```python
from build123d import *

# Parameters (mm, degrees)
F0_R     = 7.5
F1_DEPTH = 50
F3_DEPTH = 12.5
F4_W     = 15
F4_H     = 7.736891
F4_H_2   = 4.14352
F5_DEPTH = 15
F6_R     = 2
F7_DEPTH = 12.5


with BuildPart() as f1:
    # F0 (on Front) → F1 (new body)
    with BuildSketch(Plane.XZ):
        Circle(F0_R)
    extrude(amount=F1_DEPTH)

    # F2 (on Right) → F3 (cut, symmetric)
    with BuildSketch(Plane.YZ):
        Polygon((-44.571992, 11.14893), (-51.264416, 11.14893), (-51.264416, -8.581314), (-47.007408, -8.41625), (-48.95056, -5.98029), (-47.531635, -4.853975), (-43.883123, -4.709495), (-48.910081, -2.602493), (-46.984833, -0.98913), (-49.004711, 1.153992), (-42.819649, 1.551311), (-48.76826, 3.143417), (-46.388377, 4.090473), (-48.69375, 6.484859), align=None)
    extrude(amount=F3_DEPTH, both=True, mode=Mode.SUBTRACT)

    # F4 (on Front) → F5 (cut)
    with BuildSketch(Plane.XZ):
        with Locations((-0.000368, -8.868445)):
            Rectangle(F4_W, F4_H)
        with Locations((0.000368, 7.07176)):
            Rectangle(F4_W, F4_H_2)
    extrude(amount=F5_DEPTH, mode=Mode.SUBTRACT)

    # F6 (on Right) → F7 (cut, symmetric)
    with BuildSketch(Plane.YZ):
        with Locations((-7.5, 0)):
            Circle(F6_R)
    extrude(amount=F7_DEPTH, both=True, mode=Mode.SUBTRACT)


solid = f1.part
```
Build history of the part. All positions in model axes, mm. A direction names the side the tool comes from. Coordinates: 2 decimals unless noted, no trailing zeros. Order: outer loops, then holes, each group sorted by start corner. A loop starts at its lowest first (then second) coordinate and runs counter-clockwise, first axis right, second up. Notation, with made-up numbers: (38.5, 64.25) -> (93.5, 64.25) arc R31 cw to (93.5, 93.25) -> close; hole circle Ø3 at (4, 70). An arc over 180 degrees is marked (long way). Answer in a Markdown table with one row per item. Add a question column.
Q1. Band-saw the part on D-D, the plane y = -35. List the corners of the cut face in (x, z).
Q2. Which spindle directions (+Z, -Z, +X, -X, +Y, -Y) get a long thin tool onto all of the face, cutting with end or side? Do faces 5 (the face through (0, -7, -5)), 6 (the face through (0.104, -47.961, -1.807)), 7 (the face through (0.06, -48.47, -6.58)), 8 (the face through (0, -15, 6)). Say none if no direction does.
Q3. Band-saw the part on A-A, the plane x = 0. List the corners of the cut face in (y, z).
Q4. Band-saw the part on C-C, the plane z = 0. List the corners of the cut face in (x, y).
Q5. Band-saw the part on B-B, the plane y = -6.5. List the corners of the cut face in (x, z).
Q6. Drop flat-ended pins along their axis: pin 1 (3 mm diameter, centred on x = -5.5, z = 0, fed in from +Y); pin 2 (5 mm diameter, centred on y = -39, z = -5.5, fed in from +X); pin 3 (1 mm diameter, centred on x = 3.5, z = -5, fed in from -Y); pin 4 (1.5 mm diameter, centred on x = 1.5, z = -0.5, fed in from -Y). Give the stop position or say it passes through.
Q7. Wall check: line 1 along Z through (x, y) = (0.75, -7.5); line 2 along Z through (x, y) = (1, -12.5); line 3 along Z through (x, y) = (-5, -33.5). Give the ranges that are in metal, low to high. Write a range as [from, to].
Q8. Mould opens along Z. For faces 1 (the face through (0.053, -48.351, 6.873)), 2 (the face through (0.105, -9.498, 0.088)), 3 (the face through (3.461, -29.604, -6.654)), 4 (the face through (0, 0, 0)) say: +Z half, -Z half, draft (parallel to the pull), parting line (faces both ways), or undercut.
Answers follow:
| question | item | result |
|---|---|---|
| 1 | outline | circle Ø15 at (0, 0) |
| 2 | face 5 | -Z, +X, -X, +Y |
| 2 | face 6 | +X, -X, -Y |
| 2 | face 7 | -Z, +X, -X, -Y |
| 2 | face 8 | +Z, +X, -X, +Y |
| 3 | outline | (-49, 1.15) -> (-46.98, -0.99) -> (-48.91, -2.6) -> (-43.88, -4.71) -> (-47.53, -4.85) -> (-48.95, -5.98) -> (-47.74, -7.5) -> (-15, -7.5) -> (-15, -5) -> (0, -5) -> (0, 5) -> (-15, 5) -> (-15, 7.5) -> (-47.8, 7.5) -> (-48.69, 6.48) -> (-46.39, 4.09) -> (-48.77, 3.14) -> (-42.82, 1.55) -> close; hole circle Ø4 at (-7.5, 0) |
| 4 | outline | (-7.5, -47.92) -> (7.5, -47.92) -> (7.5, -9.5) -> (-7.5, -9.5) -> close; (-7.5, -5.5) -> (7.5, -5.5) -> (7.5, 0) -> (-7.5, 0) -> close |
| 5 | outline | (-7.3, -1.73) arc R7.5 ccw to (-5.59, -5) -> (5.59, -5) arc R7.5 ccw to (7.3, -1.73) -> close; (-7.3, 1.73) -> (7.3, 1.73) arc R7.5 ccw to (5.59, 5) -> (-5.59, 5) arc R7.5 ccw to start |
| 6 | pin 1 | y = 0 |
| 6 | pin 2 | x = 6.87 |
| 6 | pin 3 | y = -48.35 |
| 6 | pin 4 | y = -48.15 |
| 7 | line 1 | [-5, -2], [2, 5] |
| 7 | line 2 | [-5, 5] |
| 7 | line 3 | [-5.59, 5.59] |
| 8 | face 1 | +Z half |
| 8 | face 2 | undercut |
| 8 | face 3 | parting line |
| 8 | face 4 | draft |
